Part model, mm, in its own coordinate system. A direction names the side the tool comes from. Give positions to 0.01 mm unless a question says otherwise; leave off trailing zeros. Write each loop counter-clockwise with the first axis right and the second up, starting at its lowest first coordinate (ties: lowest second). Pieces come first, ordered by that corner, then holes. Notation, with made-up numbers: (-3.75, -15.5) - (22.25, -15.5) arc R19 cw to (22.25, 17.5) - close; hole circle Ø8 at (67, 59). An arc over 180 degrees is marked (long way). Answer as a JSON object with one key per item and string values. Group by question number.
```python
from build123d import *

# Parameters (mm, degrees)
SKETCH1_R                = 10
SKETCH1_R_2              = 5
BOSS_EXTRUDE1_DEPTH      = 5
SKETCH1_2_R              = 5
BOSS_EXTRUDE2_DEPTH      = 55
CHAMFER1_SIZE            = 3
CHAMFER1_SIZE2           = 2
BOSS_EXTRUDE3_DEPTH      = 10
BOSS_EXTRUDE3_DEPTH_BACK = 10
SKETCH2_R                = 1.25


with BuildPart() as part:
    # Sketch1 → Boss-Extrude1 (new body)
    with BuildSketch(Plane.XY):
        Circle(SKETCH1_R)
        Circle(SKETCH1_R_2, mode=Mode.SUBTRACT)
    extrude(amount=BOSS_EXTRUDE1_DEPTH)

    # Sketch1<2> → Boss-Extrude2 (add)
    with BuildSketch(Plane.XY):
        Circle(SKETCH1_2_R)
    extrude(amount=BOSS_EXTRUDE2_DEPTH)

    # Chamfer1
    chamfer1_edges = [part.edges().sort_by_distance(p)[0] for p in [
        (-10, 0, 0),
    ]]
    chamfer1_side = [part.faces().sort_by_distance(p)[0] for p in [
        (0, 0, 0),
    ]]
    chamfer(chamfer1_edges, length=CHAMFER1_SIZE, length2=CHAMFER1_SIZE2, reference=chamfer1_side[0])

    # Sketch2 → Boss-Extrude3 (add, two sides: drawn at the far end of the back side and taken through both)
    with BuildSketch(Plane(origin=(0, 0, 0), x_dir=(0, 0, -1), z_dir=(1, 0, 0)).offset(-BOSS_EXTRUDE3_DEPTH_BACK)):
        with Locations((-52, 0)):
            Circle(SKETCH2_R)
    extrude(amount=BOSS_EXTRUDE3_DEPTH + BOSS_EXTRUDE3_DEPTH_BACK)


solid = part.part
```
1) Band-saw the part on B-B (x = 0). List the corners of the cut face in (y, z).
2) Drop flat-ended pins along their axis: P1, Ø4, axis at y = -6, z = 45, coming from the +X side; P2, Ø10, axis at y = 2.5, z = 32.5, coming from the +X side; P3, Ø5, axis at y = 3, z = 10, coming from the -X side. Give the stop position or say it passes through.
3) Band-saw the part on A-A (z = 52). List the corners of the cut face in (x, y), plus the area to 3 significant figures.
4) Probe line 1 (X direction, y = 0, z = 35.5); line 2 (Z direction, x = 6.25, y = -1); line 3 (Z direction, x = 6.5, y = -1.75). List the from-to ranges inside material, lowest first.
5) Which spindle directions (+Z, -Z, +X, -X, +Y, -Y) get a long thin tool onto all of the face, cutting with end or side? Do faces 1 (the cylindrical face through (-7.46, 0.38, 50.81)), 2 (the flat face through (0, 0, 0)), 3 (the cylindrical face through (7.38, 0.38, 50.81)). Say none if no direction does.
6) Band-saw the part on D-D (z = 17.5). List the corners of the cut face in (x, y), plus the area to 3 significant figures.
7) Band-saw the part on C-C (y = 0). List the corners of the cut face in (x, z), plus the area to 3 significant figures.
Verdict:
{
 "1": {"outline": "(-10, 2) - (-7, 0) - (7, 0) - (10, 2) - (10, 5) - (5, 5) - (5, 55) - (-5, 55) - (-5, 5) - (-10, 5) - close"},
 "2": {"P1": "x = 3", "P2": "x = 5", "P3": "x = -4.97"},
 "3": {"outline": "(-10, -1.25) - (-4.84, -1.25) arc R5 ccw to (4.84, -1.25) - (10, -1.25) - (10, 1.25) - (4.84, 1.25) arc R5 ccw to (-4.84, 1.25) - (-10, 1.25) - close", "area": "104 mm2"},
 "4": {"line 1": "-5 to 5", "line 2": "0 to 5, 51.25 to 52.75", "line 3": "0 to 5"},
 "5": {"face 1": "-X", "face 2": "-Z, +X, -X, +Y, -Y", "face 3": "+X"},
 "6": {"outline": "circle Ø10 at (0, 0)", "area": "78.5 mm2"},
 "7": {"outline": "(-10, 2) - (-7, 0) - (7, 0) - (10, 2) - (10, 5) - (5, 5) - (5, 50.75) - (10, 50.75) - (10, 53.25) - (5, 53.25) - (5, 55) - (-5, 55) - (-5, 53.25) - (-10, 53.25) - (-10, 50.75) - (-5, 50.75) - (-5, 5) - (-10, 5) - close", "area": "619 mm2"}
}
